Could you check a few things on this model? Use its own coordinates, in mm. Face numbers are marked on the shaded views. Give positions to 0.01 mm unless a question says otherwise; leave off trailing zeros. Order: outer loops, then holes, each group sorted by start corner. A loop starts at its lowest first (then second) coordinate and runs counter-clockwise, first axis right, second up. Notation, with made-up numbers: M 79.5,14 L 93.5,14 A20 ccw 93.5,36 Z; hole C 21,-18.75 d11. An arc over 180 degrees is marked long. Use a Markdown table: item, result. Add a question column.
Item 1: Suppose I cut it at C-C on y = 3.5. Write out the boundary of the cut face in (x, z).
Item 2: If we mould it in two halves opening along X, with no side actions, what happens to the marked faces 1, 2 and 3? For each: released by +X, released by -X, zero draft, split by the parting line, or undercut.
Item 3: If I drill on L1, parallel to X at y = 0.3, z = 0; L2, parallel to X at y = 2.25, z = 0; L3, parallel to X at y = 5.75, z = -4, over which ranges is the centre line in solid material (lowest first)? Write a range as from..to.
Item 4: I'm going to push flat-ended pins straight in: pin 1 Ø2 at (y, z) = (3, -9.5) entering from +X; pin 2 Ø1.5 at (y, z) = (1.5, -19) entering from -X; pin 3 Ø3 at (y, z) = (2, 9.5) entering from -X. Where does each tip first touch, or does it pass through?
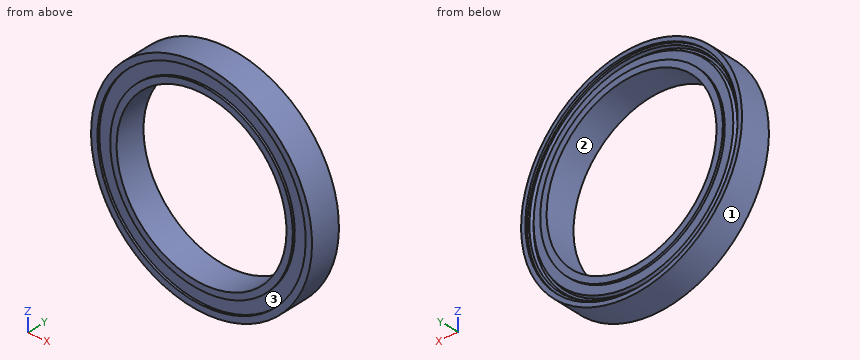
from build123d import *

# Parameters (mm, degrees)
SKETCH_1_R          = 26
SKETCH_1_R_2        = 20
EXTRUDE_1_DEPTH     = 7
SKETCH_2_R          = 25
SKETCH_2_R_2        = 21.5
CUT_EXTRUDE_1_DEPTH = 0.5
SKETCH_3_R          = 24.5
SKETCH_3_R_2        = 23.5
CUT_EXTRUDE_2_DEPTH = 0.8
CUT_EXTRUDE_2_DRAFT = -17
CUT_EXTRUDE_START   = -0.5
SKETCH_4_R          = 24.5
SKETCH_4_R_2        = 21.5
CUT_EXTRUDE_3_DEPTH = 0.5


with BuildPart() as part:
    # Эскиз1 → Бобышка-Вытянуть1 (new body)
    with BuildSketch(Plane(origin=(0, 0, 0), x_dir=(1, 0, 0), z_dir=(0, 1, 0))):
        with Locations(Location((0, 0, 0), (0, 0, 270))):
            Circle(SKETCH_1_R)
        with Locations(Location((0, 0, 0), (0, 0, 270))):
            Circle(SKETCH_1_R_2, mode=Mode.SUBTRACT)
    extrude(amount=EXTRUDE_1_DEPTH)

    # Эскиз2 → Вырез-Вытянуть1 (cut)
    with BuildSketch(Plane(origin=(0, 7, 0), x_dir=(1, 0, 0), z_dir=(0, 1, 0))):
        with Locations(Location((0, 0, 0), (0, 0, 270))):
            Circle(SKETCH_2_R)
        with Locations(Location((0, 0, 0), (0, 0, 270))):
            Circle(SKETCH_2_R_2, mode=Mode.SUBTRACT)
    extrude(amount=-CUT_EXTRUDE_1_DEPTH, mode=Mode.SUBTRACT)


with BuildPart() as cut_extrude_2_tool:
    # Эскиз3 → Вырез-Вытянуть2 (with draft: the straight prism first)
    with BuildSketch(Plane(origin=(0, 6.5, 0), x_dir=(1, 0, 0), z_dir=(0, 1, 0))):
        Circle(SKETCH_3_R)
        Circle(SKETCH_3_R_2, mode=Mode.SUBTRACT)
    extrude(amount=-CUT_EXTRUDE_2_DEPTH)
    # Вырез-Вытянуть2: the draft: its side faces are tilted about the plane it starts from
    cut_extrude_2_sides = [cut_extrude_2_tool.faces().sort_by_distance(p)[0] for p in [
        (-24.5, 6.1, 0),
        (-23.5, 6.1, 0),
    ]]
    draft(cut_extrude_2_sides, Plane(origin=(0, 6.5, 0), x_dir=(1, 0, 0), z_dir=(0, 1, 0)), CUT_EXTRUDE_2_DRAFT)


with BuildPart() as part_1:
    add(part.part)

    # Вырез-Вытянуть2: cut by cut_extrude_2_tool
    add(cut_extrude_2_tool.part, mode=Mode.SUBTRACT)

    # Эскиз4 → Вырез-Вытянуть3 (cut)
    with BuildSketch(Plane.XZ.offset(CUT_EXTRUDE_START)):
        with Locations(Location((0, 0, 0), (0, 0, 270))):
            Circle(SKETCH_4_R)
        with Locations(Location((0, 0, 0), (0, 0, 90))):
            Circle(SKETCH_4_R_2, mode=Mode.SUBTRACT)
    extrude(amount=CUT_EXTRUDE_3_DEPTH, mode=Mode.SUBTRACT)


solid = part_1.part
Findings below:
| question | item | result |
|---|---|---|
| 1 | outline | C 0,0 d52; hole C 0,0 d40 |
| 2 | face 1 | split by the parting line |
| 2 | face 2 | undercut |
| 2 | face 3 | undercut |
| 3 | L1 | x = -26..-24.5, -21.5..-20, 20..21.5, 24.5..26 |
| 3 | L2 | x = -26..-20, 20..26 |
| 3 | L3 | x = -25.69..-23.94, -23.39..-19.6, 19.6..23.39, 23.94..25.69 |
| 4 | pin 1 | stops at x = 24.57 |
| 4 | pin 2 | stops at x = -18.52 |
| 4 | pin 3 | stops at x = -24.74 |
